Check sheet for the modelled part. Datum: model origin and axes. Units: mm. A direction names the side the tool comes from. Round coordinates to 2 decimals unless told otherwise and drop trailing zeros. Order: outer loops, then holes, each group sorted by start corner. A loop starts at its lowest first (then second) coordinate and runs counter-clockwise, first axis right, second up. Notation, with made-up numbers: (4.25, -3) -> (55.25, -3) arc R25 ccw to (55.25, 34) -> close; hole circle Ø10 at (80, 8.5). An arc over 180 degrees is marked (long way). Answer in a Markdown table with one row per item.
```python
from build123d import *

# Parameters (mm, degrees)
EXTRUDE_1_DEPTH     = 50
SKETCH_2_W          = 8.5
SKETCH_2_H          = 10.5
CUT_EXTRUDE_1_DEPTH = 52.870829554
SKETCH_3_W          = 2.75
SKETCH_3_H          = 10.5
CUT_EXTRUDE_2_DEPTH = 52.870829554
SKETCH_4_R          = 1.75
CUT_EXTRUDE_3_DEPTH = 53.975575482
SKETCH_6_W          = 11.25
SKETCH_6_H          = 20
CUT_EXTRUDE_4_DEPTH = 54.255716697


with BuildPart() as part:
    # 草图1 → 凸台-拉伸1 (new body)
    with BuildSketch(Plane(origin=(0, 0, 0), x_dir=(1, 0, 0), z_dir=(0, 1, 0))):
        with BuildLine():
            Line((-8.953846154, 10.507692308), (-8.953846154, -5.492307692))
            Line((-8.953846154, -5.492307692), (3.046153846, -5.492307692))
            ThreePointArc((3.046153846, -5.492307692), (4.460367409, -4.906521255), (5.046153846, -3.492307692))
            Line((5.046153846, -3.492307692), (5.046153846, 8.507692308))
            ThreePointArc((5.046153846, 8.507692308), (4.460367409, 9.92190587), (3.046153846, 10.507692308))
            Line((3.046153846, 10.507692308), (-8.953846154, 10.507692308))
        make_face()
    extrude(amount=EXTRUDE_1_DEPTH)

    # 草图2 → 切除-拉伸1 (cut, through all)
    with BuildSketch(Plane(origin=(0, 50, 0), x_dir=(1, 0, 0), z_dir=(0, 1, 0))):
        with Locations((-1.953846154, 2.507692308)):
            Rectangle(SKETCH_2_W, SKETCH_2_H)
    extrude(amount=-CUT_EXTRUDE_1_DEPTH, mode=Mode.SUBTRACT)

    # 草图3 → 切除-拉伸2 (cut, through all)
    with BuildSketch(Plane(origin=(0, 50, 0), x_dir=(1, 0, 0), z_dir=(0, 1, 0))):
        with Locations((-7.578846154, 2.507692308)):
            Rectangle(SKETCH_3_W, SKETCH_3_H)
    extrude(amount=-CUT_EXTRUDE_2_DEPTH, mode=Mode.SUBTRACT)

    # 草图4 → 切除-拉伸3 (cut, through all)
    with BuildSketch(Plane(origin=(5.046153846, 0, 0), x_dir=(0, 0, -1), z_dir=(1, 0, 0))):
        with Locations((2.507692308, 43)):
            Circle(SKETCH_4_R)
        with Locations((2.507692308, 6)):
            Circle(SKETCH_4_R)
    extrude(amount=-CUT_EXTRUDE_3_DEPTH, mode=Mode.SUBTRACT)

    # 草图6 → 切除-拉伸4 (cut, through all)
    with BuildSketch(Plane(origin=(0, 0, -10.507692308), x_dir=(-1, 0, 0), z_dir=(0, 0, -1))):
        with Locations((3.328846154, 25)):
            Rectangle(SKETCH_6_W, SKETCH_6_H)
    extrude(amount=-CUT_EXTRUDE_4_DEPTH, mode=Mode.SUBTRACT)


solid = part.part
```
(1) Section check D-D on y = 34. Record the boundary of the cut face in (x, z).
Solutions:
| item | result |
|---|---|
| outline | (2.3, -10.51) -> (3.05, -10.51) arc R2 ccw to (5.05, -8.51) -> (5.05, 3.49) arc R2 ccw to (3.05, 5.49) -> (2.3, 5.49) -> close |
(2) Tool access check on faces 4 (the flat face through (-3, 15, 4)), 5 (the flat face through (-3, 43, -7.758)), 6 (the flat face through (3, 0, -4)). Record the directions out of +Z, -Z, +X, -X, +Y, -Y that give a thin tool (end or side, any length) a straight path to the whole face; none if there is none.
Solutions:
| item | result |
|---|---|
| face 4 | +Z, -Z, -X |
| face 5 | -X, +Y, -Y |
| face 6 | +Z, -Z, +X, -X, -Y |
(3) Depth check by flat-ended pin: pin 1 Ø3 at (x, z) = (-4.5, 3.5) entering from -Y; pin 2 Ø3 at (y, z) = (43, -2.51) entering from -X; pin 3 Ø8 at (y, z) = (17, -3) entering from -X. Enter the tip coordinate at first touch or a pass-through.
Solutions:
| item | result |
|---|---|
| pin 1 | y = 0 |
| pin 2 | through |
| pin 3 | x = 2.3 |
(4) Draft check along Z on faces 1 (the flat face through (3, 50, -4)), 2 (the flat face through (2.296, 25, -2)), 3 (the flat face through (2.5, 24.6, -10.508)). Enter one of: pulls with the +Z half, pulls with the -Z half, needs draft (parallel to the pull), parting line crosses it, or undercut.
Solutions:
| item | result |
|---|---|
| face 1 | needs draft |
| face 2 | undercut |
| face 3 | pulls with the -Z half |
(5) Section check A-A on y = 43. Record the boundary of the cut face in (x, z).
Solutions:
| item | result |
|---|---|
| outline | (-8.95, -10.51) -> (3.05, -10.51) arc R2 ccw to (5.05, -8.51) -> (5.05, -4.26) -> (2.3, -4.26) -> (2.3, -7.76) -> (-8.95, -7.76) -> close; (-8.95, 2.74) -> (2.3, 2.74) -> (2.3, -0.76) -> (5.05, -0.76) -> (5.05, 3.49) arc R2 ccw to (3.05, 5.49) -> (-8.95, 5.49) -> close |
(6) Section check B-B on x = -1. Record the boundary of the cut face in (y, z), plus the area to 3 significant figures.
Solutions:
| item | result |
|---|---|
| outline | (0, -10.51) -> (15, -10.51) -> (15, -7.76) -> (0, -7.76) -> close; (0, 2.74) -> (15, 2.74) -> (15, 5.49) -> (0, 5.49) -> close; (35, -10.51) -> (50, -10.51) -> (50, -7.76) -> (35, -7.76) -> close; (35, 2.74) -> (50, 2.74) -> (50, 5.49) -> (35, 5.49) -> close |
| area | 165 mm^2 |
(7) Section check C-C on z = -1.75. Record the boundary of the cut face in (x, y).
Solutions:
| item | result |
|---|---|
| outline | (2.3, 0) -> (5.05, 0) -> (5.05, 4.42) -> (2.3, 4.42) -> close; (2.3, 7.58) -> (5.05, 7.58) -> (5.05, 41.42) -> (2.3, 41.42) -> close; (2.3, 44.58) -> (5.05, 44.58) -> (5.05, 50) -> (2.3, 50) -> close |
(8) Scan lines: probe 1 along Z at (x, y) = (1, 37); probe 2 along Y at (x, z) = (-3, -8.25); probe 3 along X at (y, z) = (30.5, -6.5). Record each from-to range of solid material in increasing order. Write a range as from..to.
Solutions:
| item | result |
|---|---|
| probe 1 | -10.51..-7.76, 2.74..5.49 |
| probe 2 | 0..15, 35..50 |
| probe 3 | 2.3..5.05 |
